```python
from build123d import *

# Parameters (mm, degrees)
SCHIZZO1_R               = 12.5
ESTRUSIONE1_DEPTH        = 569
SCHIZZO2_R               = 7
ESTRUSIONE2_DEPTH        = 64.5
SCHIZZO3_R               = 3
TAGLIO_ESTRUSIONE1_DEPTH = 20
TAGLIO_ESTRUSIONE2_START = -20
SCHIZZO4_R               = 3
TAGLIO_ESTRUSIONE2_DEPTH = 20
SCHIZZO5_R               = 40
ESTRUSIONE3_DEPTH        = 500
SMUSSO1_SIZE             = 2
SMUSSO2_SIZE             = 0.5
TAGLIO_ESTRUSIONE3_START = -52
TAGLIO_ESTRUSIONE3_DEPTH = 52
TAGLIO_ESTRUSIONE4_DEPTH = 10


with BuildPart() as part:
    # Schizzo1 → Estrusione1 (new body)
    with BuildSketch(Plane(origin=(0, 0, 0), x_dir=(0, 0, -1), z_dir=(1, 0, 0))):
        Circle(SCHIZZO1_R)
    extrude(amount=ESTRUSIONE1_DEPTH)

    # Schizzo2 → Estrusione2 (add)
    with BuildSketch(Plane(origin=(569, 0, 0), x_dir=(0, 0, -1), z_dir=(1, 0, 0))):
        Circle(SCHIZZO2_R)
    extrude(amount=ESTRUSIONE2_DEPTH)

    # Schizzo3 → Taglio-Estrusione1 (cut)
    with BuildSketch(Plane(origin=(633.5, 0, 0), x_dir=(0, 0, -1), z_dir=(1, 0, 0))):
        Circle(SCHIZZO3_R)
    extrude(amount=-TAGLIO_ESTRUSIONE1_DEPTH, mode=Mode.SUBTRACT)

    # Schizzo4 → Taglio-Estrusione2 (cut)
    with BuildSketch(Plane.ZY.offset(TAGLIO_ESTRUSIONE2_START)):
        with Locations(Location((0, 0, 0), (0, 0, 180))):
            Circle(SCHIZZO4_R)
    extrude(amount=TAGLIO_ESTRUSIONE2_DEPTH, mode=Mode.SUBTRACT)

    # Schizzo5 → Estrusione3 (add)
    with BuildSketch(Plane.ZY.offset(-34)):
        Circle(SCHIZZO5_R)
    extrude(amount=-ESTRUSIONE3_DEPTH)

    # Smusso1
    smusso1_edges = [part.edges().sort_by_distance(p)[0] for p in [
        (534, 0, 12.5),
        (34, 0, 12.5),
        (569, 0, 7),
    ]]
    chamfer(smusso1_edges, length=SMUSSO1_SIZE)

    # Smusso2
    smusso2_edges = [part.edges().sort_by_distance(p)[0] for p in [
        (0, 0, 12.5),
        (569, 0, 12.5),
        (633.5, 0, 7),
    ]]
    chamfer(smusso2_edges, length=SMUSSO2_SIZE)

    # Schizzo7 → Taglio-Estrusione3 (cut)
    with BuildSketch(Plane(origin=(633.5, 0, 0), x_dir=(0, 0, -1), z_dir=(1, 0, 0)).offset(TAGLIO_ESTRUSIONE3_START)):
        with BuildLine():
            Line((-2.5, 6.538348415), (-2.5, 3.65))
            Line((-2.5, 3.65), (2.5, 3.65))
            Line((2.5, 3.65), (2.5, 6.538348415))
            ThreePointArc((2.5, 6.538348415), (0, 7), (-2.5, 6.538348415))
        make_face()
    extrude(amount=TAGLIO_ESTRUSIONE3_DEPTH, mode=Mode.SUBTRACT)

    # Schizzo8 → Taglio-Estrusione4 (cut)
    with BuildSketch(Plane(origin=(0, 3.65, 0), x_dir=(1, 0, 0), z_dir=(0, 1, 0))):
        with BuildLine():
            Line((581.5, -2.5), (581.5, 2.5))
            ThreePointArc((581.5, 2.5), (579, 0), (581.5, -2.5))
        make_face()
    extrude(amount=TAGLIO_ESTRUSIONE4_DEPTH, mode=Mode.SUBTRACT)


solid = part.part
```
Work out the finished part from the listing and answer in its coordinate system (mm). A direction names the side the tool comes from. Coordinates: 2 decimals unless noted, no trailing zeros. Loops run counter-clockwise (first coordinate to the right, second up) from the corner with the lowest first, then second, coordinate; pieces in that order, holes last. Notation, with made-up numbers: (13, 37.25) -> (29, 37.25) arc R35 cw to (29, 71.25) -> close; hole circle Ø10 at (-0.5, -6.75). An arc over 180 degrees is marked (long way). Answer as CSV lines item,"result".
Q1. The part is cut by section C-C on y = -25.5. Write down the section's boundary in (x, z), and give its area (3 significant figures).
Findings:
outline,"(34, -30.82) -> (534, -30.82) -> (534, 30.82) -> (34, 30.82) -> close"
area,"30,800 mm²"
Q2. The part is cut by section A-A on x = 171. Write down the section's boundary in (y, z).
Findings:
outline,"circle Ø80 at (0, 0)"
Q3. Each of these flat-tipped pins is pushed along its axis until it touches: pin 1 (1.5 mm diameter, centred on x = 616, z = -0.5, fed in from +Y); pin 2 (2 mm diameter, centred on y = -8, z = -22, fed in from +X); pin 3 (1.5 mm diameter, centred on x = 520.5, z = -28, fed in from +Y). Where does it stop, or does it pass through?
Findings:
pin 1,"stops at y = 3.65"
pin 2,"stops at x = 534"
pin 3,"stops at y = 29.28"
Q4. Find the intervals of material crossed by probe 1 along Y at (x, z) = (7, 0); probe 2 along X at (y, z) = (-11.5, -3.5); probe 3 along X at (y, z) = (-2, -16), in increasing order.
Findings:
probe 1,"y = -12.5 to -3, 3 to 12.5"
probe 2,"x = 0.02 to 568.98"
probe 3,"x = 34 to 534"
Q5. A tool of negligible diameter and unlimited length cuts with its end or side. For faces 1 (the face through (534, -17, -1)), 2 (the face through (34, -17, -1)), 3 (the face through (633.5, -3, -1)), from which of +Z, -Z, +X, -X, +Y, -Y can it reach the whole face along a straight path? Write none if from no direction.
Findings:
face 1,"+X"
face 2,"-X"
face 3,"+Z, -Z, +X, +Y, -Y"
Q6. The part is cut by section B-B on z = -20. Write down the section's boundary in (x, y), and give its area (3 significant figures).
Findings:
outline,"(34, -34.64) -> (534, -34.64) -> (534, 34.64) -> (34, 34.64) -> close"
area,"34,600 mm²"
